The listing builds one solid part. Answer for the finished solid, in the listing's coordinates (mm). Coordinates: 2 decimals unless noted, no trailing zeros. Order: outer loops, then holes, each group sorted by start corner. A loop starts at its lowest first (then second) coordinate and runs counter-clockwise, first axis right, second up.
from build123d import *

# Parameters (mm, degrees)
SKETCH1_W           = 500
SKETCH1_H           = 1000
BOSS_EXTRUDE1_DEPTH = 100
SKETCH2_R           = 15
CUT_EXTRUDE1_DEPTH  = 501
FILLET1_R           = 80
FILLET2_R           = 10


with BuildPart() as part:
    # Sketch1 → Boss-Extrude1 (new body)
    with BuildSketch(Plane(origin=(0, 0, 0), x_dir=(1, 0, 0), z_dir=(0, 1, 0))):
        with Locations((250, -500)):
            Rectangle(SKETCH1_W, SKETCH1_H)
    extrude(amount=BOSS_EXTRUDE1_DEPTH)

    # Sketch2 → Cut-Extrude1 (cut, through all)
    with BuildSketch(Plane(origin=(500, 0, 0), x_dir=(0, 0, -1), z_dir=(1, 0, 0))):
        with Locations((-850, 47.419401297)):
            Circle(SKETCH2_R)
        with Locations((-150, 47.419401297)):
            Circle(SKETCH2_R)
    extrude(amount=-CUT_EXTRUDE1_DEPTH, mode=Mode.SUBTRACT)

    # Fillet1
    fillet1_edges = [part.edges().sort_by_distance(p)[0] for p in [
        (0, 50, 0),
        (500, 50, 0),
    ]]
    fillet(fillet1_edges, radius=FILLET1_R)

    # Fillet2
    fillet2_edges = [part.edges().sort_by_distance(p)[0] for p in [
        (500, 100, 540),
        (250, 100, 0),
        (0, 100, 540),
        (23.431457505, 100, 23.431457505),
        (476.568542495, 100, 23.431457505),
    ]]
    fillet(fillet2_edges, radius=FILLET2_R)


solid = part.part
(1) The mould has two halves that part along Y. Classify faces 1 (the flat face through (247, 100, 498)), 2 (the cylindrical face through (253.5, 41.674, 836.144)), 3 (the cylindrical face through (475.94, 45.63, 22.81)): pulls with the +Y half, pulls with the -Y half, needs draft (parallel to the pull), parting line crosses it, or undercut.
(2) Find section A-A on z = 850. Determine the outline of the cut face in (x, y), then the cut area to 3 significant figures.
(3) Find section C-C on x = 469. Count the separate pieces of the cut face and the enclosed holes in it, then the cut area to 3 significant figures.
(4) Find the intervals of material crossed by probe 1 along Y at (x, z) = (181, 850); probe 2 along Z at (x, y) = (178.5, 51.5); probe 3 along Z at (x, y) = (366.5, 92), in increasing order.
(5) Find section B-B on z = 155. Determine the outline of the cut face in (x, y), then the cut area to 3 significant figures.
Resolved:
1. face 1: pulls with the +Y half
1. face 2: undercut
1. face 3: needs draft
2. outline: (0, 0) - (500, 0) - (500, 32.42) - (0, 32.42) - close; (0, 62.42) - (500, 62.42) - (500, 90) arc R10 ccw to (490, 100) - (10, 100) arc R10 ccw to (0, 90) - close
2. area: 35,000 mm2
3. separate pieces: 1
3. enclosed holes: 2
3. area: 96,900 mm2
4. probe 1: y = 0 to 32.42, 62.42 to 100
4. probe 2: z = 0 to 135.57, 164.43 to 835.57, 864.43 to 1000
4. probe 3: z = 0.2 to 1000
5. outline: (0, 0) - (500, 0) - (500, 33.28) - (0, 33.28) - close; (0, 61.56) - (500, 61.56) - (500, 90) arc R10 ccw to (490, 100) - (10, 100) arc R10 ccw to (0, 90) - close
5. area: 35,800 mm2
